from build123d import *

# Parameters (mm, degrees)
SKETCH2_R           = 9.652
BOSS_EXTRUDE1_DEPTH = 63.5
CHAMFER1_SIZE       = 1.27
BOSS_EXTRUDE2_DEPTH = 2.54
CHAMFER2_SIZE       = 0.508
FILLET1_R           = 5.08
SKETCH7_R           = 5.08
CUT_EXTRUDE1_DEPTH  = 1.27
CUT_EXTRUDE1_DRAFT  = -20
FILLET2_R           = 1.27


with BuildPart() as part:
    # Sketch2 → Boss-Extrude1 (new body)
    with BuildSketch(Plane(origin=(0, 0, 0), x_dir=(1, 0, 0), z_dir=(0, 1, 0))):
        with Locations(Location((0, 0, 0), (0, 0, 270))):
            Circle(SKETCH2_R)
    extrude(amount=BOSS_EXTRUDE1_DEPTH)

    # Chamfer1
    chamfer1_edges = [part.edges().sort_by_distance(p)[0] for p in [
        (0, 0, -9.652),
    ]]
    chamfer(chamfer1_edges, length=CHAMFER1_SIZE)

    # Sketch6 → Boss-Extrude2 (add, symmetric)
    with BuildSketch(Plane(origin=(0, 63.5, 0), x_dir=(1, 0, 0), z_dir=(0, 1, 0))):
        Polygon((0, 15.24), (-13.198227154, 7.62), (-13.198227154, -7.62), (0, -15.24), (13.198227154, -7.62), (13.198227154, 7.62), align=None)
    extrude(amount=BOSS_EXTRUDE2_DEPTH, both=True)

    # Chamfer2
    chamfer2_edges = [part.edges().sort_by_distance(p)[0] for p in [
        (-13.198227154, 60.96, 0),
        (-6.599113577, 60.96, 11.43),
        (6.599113577, 60.96, 11.43),
        (13.198227154, 60.96, 0),
        (6.599113577, 66.04, -11.43),
        (-6.599113577, 66.04, -11.43),
        (-13.198227154, 66.04, 0),
        (-6.599113577, 66.04, 11.43),
        (6.599113577, 66.04, 11.43),
        (13.198227154, 66.04, 0),
        (6.599113577, 60.96, -11.43),
        (-6.599113577, 60.96, -11.43),
    ]]
    chamfer(chamfer2_edges, length=CHAMFER2_SIZE)

    # Fillet1
    # the kernel refuses this fillet: 5.08 mm, written as the material it takes off along each edge
    with BuildSketch(Plane(origin=(-13.198227154, 54.135651581, -7.62), x_dir=(0, 0, 1), z_dir=(0, 1, 0)), Plane(origin=(13.198227154, 72.864348419, 7.62), x_dir=(-0.8660254037844387, 0, 0.5), z_dir=(0, -1, 0))) as fillet1_piece_1:
        with BuildLine():
            CenterArc((FILLET1_R * 0.57735026919, FILLET1_R), FILLET1_R, 210, 60)
            Line((-FILLET1_R * 0.288675134595, FILLET1_R * 0.5), (0, 0))
            Line((0, 0), (FILLET1_R * 0.57735026919, 0))
        make_face()
    extrude(amount=18.728696837, mode=Mode.SUBTRACT)
    with BuildSketch(Plane(origin=(-13.198227154, 54.135651581, 7.62), x_dir=(0, 0, -1), z_dir=(0, 1, 0)), Plane(origin=(0, 72.864348419, -15.24), x_dir=(-0.8660254037844386, 0, 0.5), z_dir=(0, -1, 0)), Plane(origin=(13.198227154, 72.864348419, -7.62), x_dir=(-0.8660254037844388, 0, -0.4999999999999998), z_dir=(0, -1, 0)), Plane(origin=(0, 54.135651581, 15.24), x_dir=(-0.8660254037844386, 0, -0.5000000000000001), z_dir=(0, 1, 0))) as fillet1_piece_2:
        with BuildLine():
            CenterArc((FILLET1_R * 0.57735026919, -FILLET1_R), FILLET1_R, 90, 60)
            Line((-FILLET1_R * 0.288675134595, -FILLET1_R * 0.5), (0, 0))
            Line((0, 0), (FILLET1_R * 0.57735026919, 0))
        make_face()
    extrude(amount=18.728696837, mode=Mode.SUBTRACT)


with BuildPart() as cut_extrude1_tool:
    # Sketch7 → Cut-Extrude1 (with draft: the straight prism first)
    with BuildSketch(Plane(origin=(0, 66.04, 0), x_dir=(1, 0, 0), z_dir=(0, 1, 0))):
        Circle(SKETCH7_R)
    extrude(amount=-CUT_EXTRUDE1_DEPTH)
    # Cut-Extrude1: the draft: its side faces are tilted about the plane it starts from
    cut_extrude1_sides = [cut_extrude1_tool.faces().sort_by_distance(p)[0] for p in [
        (-5.08, 65.405, 0),
    ]]
    draft(cut_extrude1_sides, Plane(origin=(0, 66.04, 0), x_dir=(1, 0, 0), z_dir=(0, 1, 0)), CUT_EXTRUDE1_DRAFT)


with BuildPart() as part_1:
    add(part.part)

    # Cut-Extrude1: cut by cut_extrude1_tool
    add(cut_extrude1_tool.part, mode=Mode.SUBTRACT)

    # Fillet2
    fillet2_edges = [part_1.edges().sort_by_distance(p)[0] for p in [
        (-5.08, 66.04, 0),
    ]]
    fillet(fillet2_edges, radius=FILLET2_R)


solid = part_1.part
Work out the finished part from the listing and answer in its coordinate system (mm). A direction names the side the tool comes from. Coordinates: 2 decimals unless noted, no trailing zeros. Loops run counter-clockwise (first coordinate to the right, second up) from the corner with the lowest first, then second, coordinate; pieces in that order, holes last. Notation, with made-up numbers: (-18, -37.5) -> (33, -37.5) arc R22 cw to (33, -31.5) -> close; hole circle Ø1 at (49.25, -33.75). An arc over 180 degrees is marked (long way). Write each question's results on one line, items separated by ' | '. Start each with the question number.
1) For faces 1 (the cylindrical face through (-5.87, 30.7, -7.66)), 2 (the flat face through (-0.2, 66.04, 6.2)), determine the directions among +Z, -Z, +X, -X, +Y, -Y from which every point of the face is accessible in a straight line to the end or side of a thin tool.
2) Flat-ended cylindrical pins translate along their axes: P1, Ø1, axis at x = -3.5, y = 17, coming from the -Z side; P2, Ø1, axis at x = -8.5, z = -4, coming from the -Y side; P3, Ø6, axis at x = 0, y = 42, coming from the +Z side; P4, Ø12, axis at x = 2, y = 56.5, coming from the +Z side. Find the tip coordinate at first contact, or state that the pin passes through.
3) Find section A-A on z = 0. Determine the outline of the cut face in (x, y), then the cut area to 3 significant figures.
4) Find section C-C on y = 39.5. Determine the outline of the cut face in (x, z), then the cut area to 3 significant figures.
5) Consider line 1 along Y through (x, z) = (-5.25, 11.25); line 2 along Y through (x, z) = (0, 4); line 3 along Z through (x, y) = (0, 49.5). Determine where each line is inside the solid, lowest interval first.
6) Find section B-B on x = -11.5. Determine the outline of the cut face in (y, z).
Response values:
1) face 1: -Y | face 2: +Z, -Z, +X, -X, +Y
2) P1: stops at z = -9.17 | P2: stops at y = 0.51 | P3: stops at z = 9.65 | P4: stops at z = 14.45
3) outline: (-13.2, 61.47) -> (-12.69, 60.96) -> (-9.65, 60.96) -> (-9.65, 1.27) -> (-8.38, 0) -> (8.38, 0) -> (9.65, 1.27) -> (9.65, 60.96) -> (12.69, 60.96) -> (13.2, 61.47) -> (13.2, 65.53) -> (12.69, 66.04) -> (5.97, 66.04) arc R1.27 ccw to (4.78, 65.2) -> (4.62, 64.77) -> (-4.62, 64.77) -> (-4.78, 65.2) arc R1.27 ccw to (-5.97, 66.04) -> (-12.69, 66.04) -> (-13.2, 65.53) -> close | area: 1,300 mm^2
4) outline: circle Ø19.3 at (0, 0) | area: 293 mm^2
5) line 1: y = 60.96 to 66.04 | line 2: y = 0 to 64.77 | line 3: z = -9.65 to 9.65
6) outline: (60.96, -8.01) -> (61.36, -8.48) -> (65.64, -8.48) -> (66.04, -8.01) -> (66.04, 8.01) -> (65.64, 8.48) -> (61.36, 8.48) -> (60.96, 8.01) -> close
